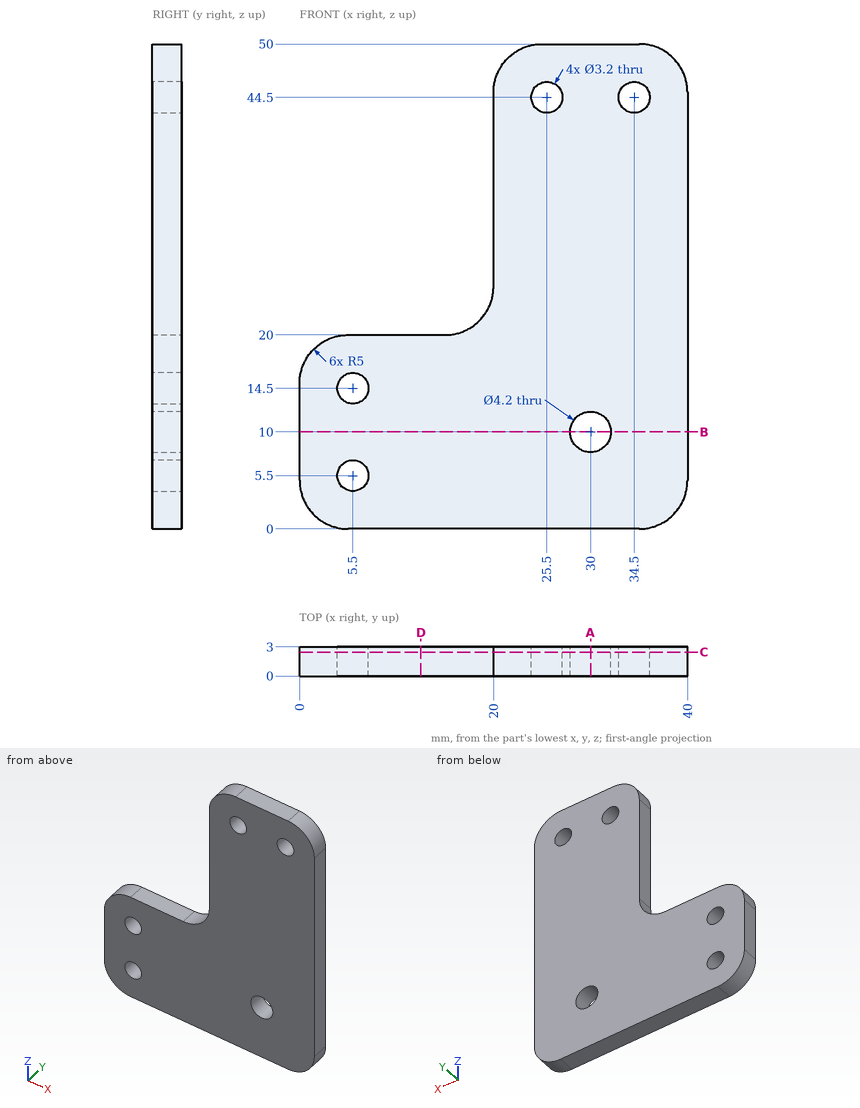
Input: dimensioned drawing with shaded views. Units: mm. Origin: part minimum x, y, z. Give positions to 0.01 mm unless a question says otherwise; leave off trailing zeros. Loops run counter-clockwise (first coordinate to the right, second up) from the corner with the lowest first, then second, coordinate; pieces in that order, holes last. Notation, with made-up numbers: M 55,53.5 L 69,53.5 A23 ccw 69,79.5 Z; hole C 56,47 d11. An arc over 180 degrees is marked long. Put each result on its own line as item: value. Start each with the question number.
1) Ray query, line 1 along X through (y, z) = (1.6, 44.5); line 2 along X through (y, z) = (1.6, 10); line 3 along X through (y, z) = (0.95, 14.5). Return the intervals inside material, ascending.
2) Cut plane D-D (x = 12.5). Output: boundary loops of the cut face in (y, z), then the cut area to 3 significant figures.
3) Contact query for flat-ended pins moving along their axis: pin 1 (1.5 mm diameter, centred on x = 9, y = 2, fed in from +Z); pin 2 (2.5 mm diameter, centred on x = 5.5, z = 5.5, fed in from -Y); pin 3 (1.5 mm diameter, centred on x = 18, y = 2.5, fed in from +Z). Output: stop coordinate, or through.
4) Cut plane C-C (y = 2.45). Output: boundary loops of the cut face in (x, z), then the cut area to 3 significant figures.
5) Cut plane A-A (x = 30). Output: boundary loops of the cut face in (y, z), then the cut area to 3 significant figures.
6) Cut plane B-B (z = 10). Output: boundary loops of the cut face in (x, y).
Verdict:
1. line 1: 20 to 23.9, 27.1 to 32.9, 36.1 to 40
1. line 2: 0 to 27.9, 32.1 to 40
1. line 3: 0 to 3.9, 7.1 to 40
2. outline: M 0,0 L 3,0 L 3,20 L 0,20 Z
2. area: 60.0 mm2
3. pin 1: z = 20
3. pin 2: through
3. pin 3: z = 21.69
4. outline: M 0,5 A5 ccw 5,0 L 35,0 A5 ccw 40,5 L 40,45 A5 ccw 35,50 L 25,50 A5 ccw 20,45 L 20,25 A5 cw 15,20 L 5,20 A5 ccw 0,15 Z; hole C 5.5,5.5 d3.2; hole C 5.5,14.5 d3.2; hole C 25.5,44.5 d3.2; hole C 30,10 d4.2; hole C 34.5,44.5 d3.2
4. area: 1,330 mm2
5. outline: M 0,0 L 3,0 L 3,7.9 L 0,7.9 Z; M 0,12.1 L 3,12.1 L 3,50 L 0,50 Z
5. area: 137 mm2
6. outline: M 0,0 L 27.9,0 L 27.9,3 L 0,3 Z; M 32.1,0 L 40,0 L 40,3 L 32.1,3 Z
